CAD build for the part. Positions are in the model's coordinates, mm. Face numbers are marked on the shaded views. A direction names the side the tool comes from. Round coordinates to 2 decimals unless told otherwise and drop trailing zeros. Loops run counter-clockwise (first coordinate to the right, second up) from the corner with the lowest first, then second, coordinate; pieces in that order, holes last.
Autodesk Inventor part; units mm, degrees
ref_plane "YZ Plane" through (0, 0, 0) normal (1, 0, 0) x (0, 1, 0)
ref_plane "XZ Plane" through (0, 0, 0) normal (0, 1, 0) x (-1, 0, 0)
ref_plane "XY Plane" through (0, 0, 0) normal (0, 0, 1) x (1, 0, 0)
sketch "Sketch1" plane through (0, 0, 0) normal (0, 0, 1) x (1, 0, 0)
  line L0 (0, 0) -> (1737.5, 0)
  line L1 (1737.5, 0) -> (1737.5, 790)
  line L2 (1737.5, 790) -> (0, 790)
  line L3 (0, 790) -> (0, 0)
  dimension "ancho" = 1737.5
  dimension "d1" = 790
extrude "Extrusion1" add sketch "Sketch1" along normal blind 50
fillet "Fillet1" radius 50 1 edges at (868.75, 0, 50)
sketch "Sketch2" plane through (1737.5, 790, 50) normal (1, 0, 0) x (0, 0, -1)
  line L0 (50, 0) -> (-50, 0)
  line L1 (-50, 0) -> (-50, 0)
  line L2 (-30, -20) -> (50, -20)
  line L3 (50, -20) -> (50, 0)
  arc A0 (-50, 0) -> (-30, -20) centre (-30, 0) ccw
  point P0 (50, -790)
  point P1 (-50, -20)
  dimension "d5" = 100
  dimension "d6" = 20
  dimension "d7" = 20
extrude "Extrusion2" add sketch "Sketch2" against normal up to surface (1737.5 mm away)
properties part number "meson"
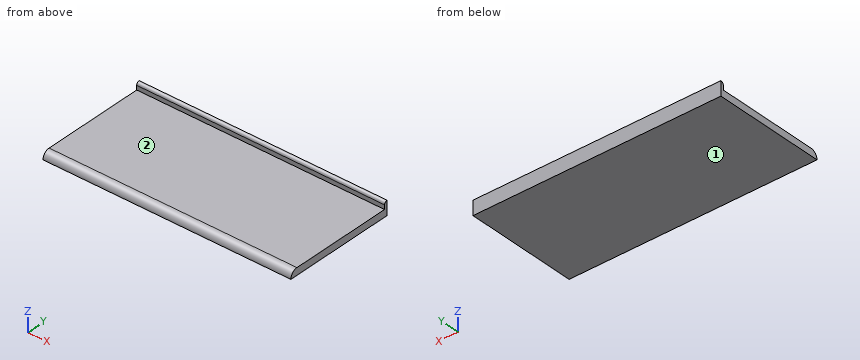
Item 1: Flat gauge pins, fed straight in: P1, Ø15, axis at x = 564, z = 59, coming from the -Y side; P2, Ø12, axis at x = 904, y = 410, coming from the +Z side. Where does each tip first touch, or does it go through?
Answers follow:
P1: stops at y = 770
P2: stops at z = 50
Item 2: 3-axis set-ups, long thin cutter, end or side, ignore diameter. For the marked faces 1 and 2: which of +Z, -Z, +X, -X, +Y, -Y reach the whole face in a straight line?
Answers follow:
face 1: -Z, +X, -X, +Y, -Y
face 2: +Z, +X, -X, -Y
Item 3: Cut at B-B, the plane y = 483. Give the cut face in (x, z), plus the area to 3 significant figures.
Answers follow:
outline: (0, 0) - (1737.5, 0) - (1737.5, 50) - (0, 50) - close
area: 86,900 mm2
Item 4: Probe line 1 (Z direction, x = 535, y = 121.5); line 2 (Y direction, x = 183.5, z = 76.5); line 3 (Y direction, x = 1374.5, z = 93.5). List the from-to ranges inside material, lowest first.
Answers follow:
line 1: z = 0 to 50
line 2: y = 770 to 790
line 3: y = 775.24 to 790
